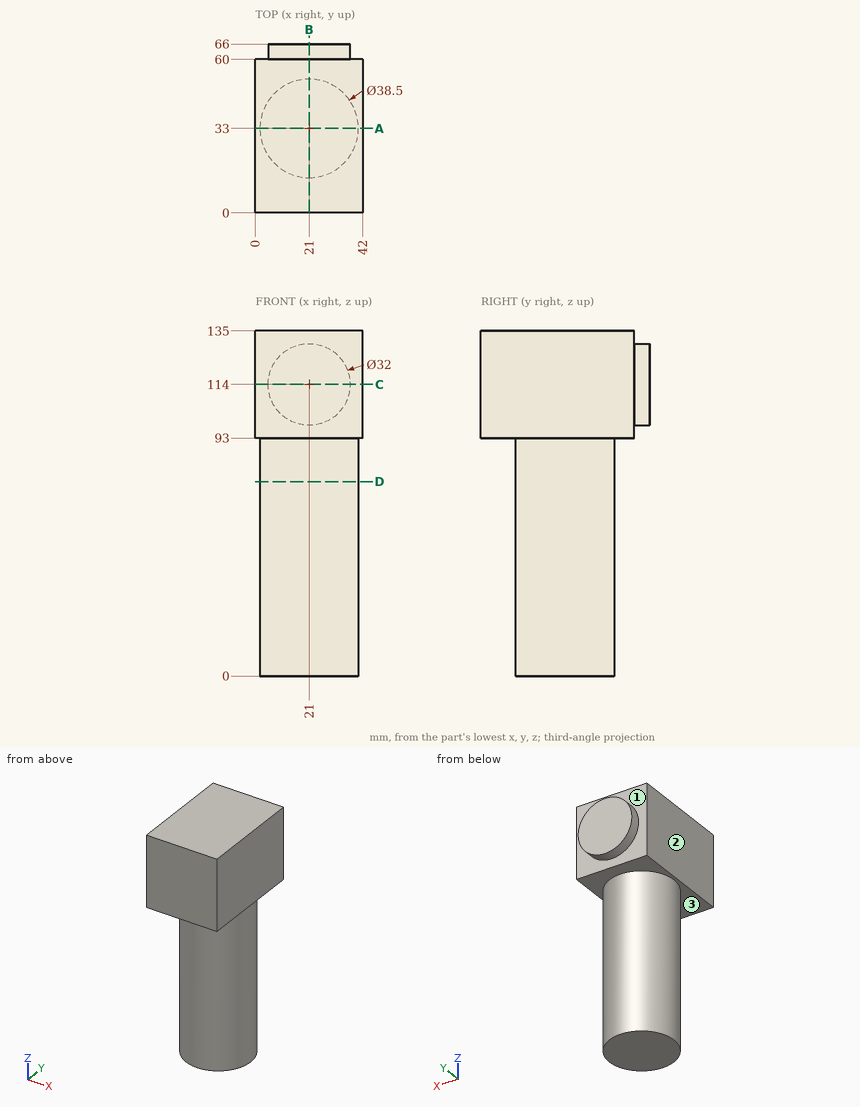
Design review of the part shown in the three views and the two pictorial views. Dimensions are in mm from the part's minimum x, y and z. A direction names the side the tool comes from. Round coordinates to 2 decimals unless told otherwise and drop trailing zeros. Write each loop counter-clockwise with the first axis right and the second up, starting at its lowest first coordinate (ties: lowest second). Pieces come first, ordered by that corner, then holes.
Item 1: For the marked faces 1, 2 and 3, list the 3-axis set-ups (+Z, -Z, +X, -X, +Y, -Y) from which the entire face can be reached by the end or side of a thin tool; tool diameter is ignored.
Item 2: Consider section B-B on x = 21. Give the boundary of the cut face in (y, z), and give its area (3 significant figures).
Item 3: Consider section A-A on y = 33. Give the boundary of the cut face in (x, z).
Item 4: Consider section D-D on z = 76. Give the boundary of the cut face in (x, y).
Item 5: For pin 1 Ø5 at (x, z) = (26, 70) entering from -Y; pin 2 Ø4 at (x, z) = (18.5, 49.5) entering from -Y; pin 3 Ø4 at (y, z) = (46.5, 39.5) entering from +X, all flat-tipped, find the tip position at first contact; note any pin that passes through.
Item 6: Consider section C-C on z = 114. Give the boundary of the cut face in (x, y), and give its area (3 significant figures).
Item 7: Wall thickness on L1, parallel to Z at x = 6, y = 11.5; L2, parallel to Y at x = 21.5, z = 56; L3, parallel to X at y = 31, z = 51.5: over which ranges is each line inside the solid? List them lowest first.
Check values:
1. face 1: +Y
1. face 2: +Z, -Z, -X, +Y, -Y
1. face 3: -Z
2. outline: (0, 93) - (13.75, 93) - (13.75, 0) - (52.25, 0) - (52.25, 93) - (60, 93) - (60, 98) - (66, 98) - (66, 130) - (60, 130) - (60, 135) - (0, 135) - close
2. area: 6,290 mm2
3. outline: (0, 93) - (1.75, 93) - (1.75, 0) - (40.25, 0) - (40.25, 93) - (42, 93) - (42, 135) - (0, 135) - close
4. outline: circle Ø38.5 at (21, 33)
5. pin 1: stops at y = 13.91
5. pin 2: stops at y = 13.76
5. pin 3: stops at x = 36.44
6. outline: (0, 0) - (42, 0) - (42, 60) - (37, 60) - (37, 66) - (5, 66) - (5, 60) - (0, 60) - close
6. area: 2,710 mm2
7. L1: z = 93 to 135
7. L2: y = 13.76 to 52.24
7. L3: x = 1.85 to 40.15
